Could you check a few things on this drawing? It's one solid part, dimensions in mm from its lowest x, y, z. A direction names the side the tool comes from. Give positions to 0.01 mm unless a question says otherwise; leave off trailing zeros. Loops run counter-clockwise (first coordinate to the right, second up) from the corner with the lowest first, then second, coordinate; pieces in that order, holes last. Notation, with made-up numbers: (76.25, -40) -> (127.25, -40) arc R22 cw to (127.25, -13) -> close; hole circle Ø4 at (28, -11). An arc over 180 degrees is marked (long way). One line per question, with ' | ' between items.
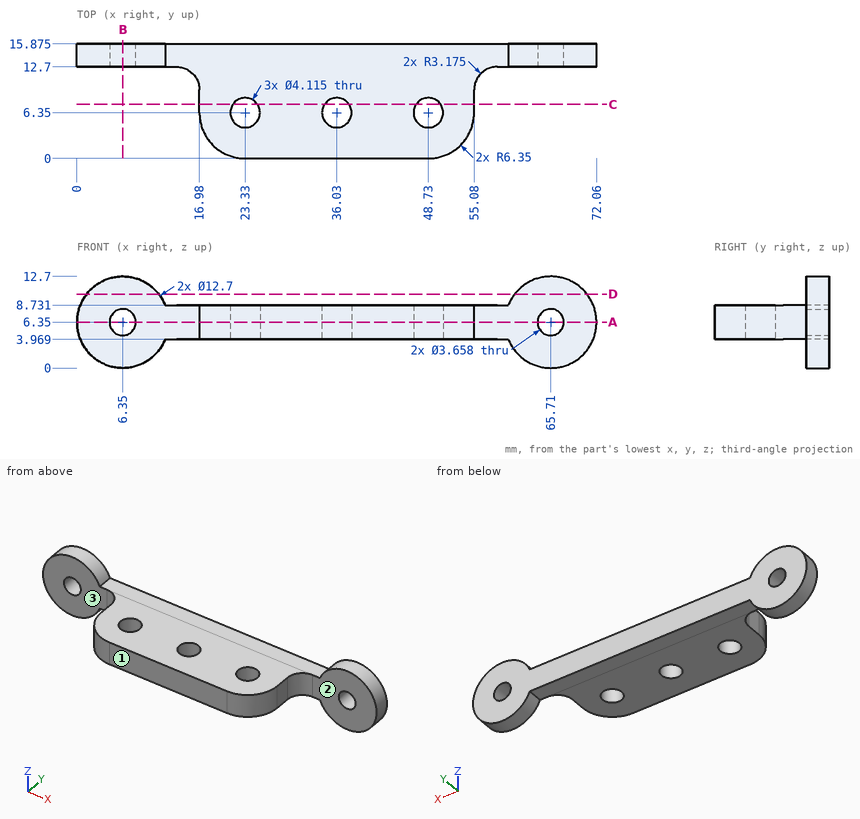
Q1. For pin 1 Ø6 at (x, z) = (61.5, 8) entering from -Y; pin 2 Ø2.5 at (x, y) = (29, 14.5) entering from +Z; pin 3 Ø1.6 at (x, y) = (28, 15) entering from -Z; pin 4 Ø6 at (x, z) = (65.71, 6.35) entering from +Y (3 decimals), each with a flat end and sliding along its axis, tell me the tip position at first contact or that it passes through.
Entries:
pin 1: y = 12.7 | pin 2: z = 8.73 | pin 3: z = 3.97 | pin 4: y = 15.875
Q2. If we section it at B-B (x = 6.35): Write out the boundary of the cut face in (y, z) (1 decimal).
Entries:
outline: (12.7, 0) -> (15.9, 0) -> (15.9, 4.5) -> (12.7, 4.5) -> close; (12.7, 8.2) -> (15.9, 8.2) -> (15.9, 12.7) -> (12.7, 12.7) -> close
Q3. On a 3-axis mill with a long thin cutter (end or side, diameter ignored), from which of +Z, -Z, +X, -X, +Y, -Y can I reach the whole of each face in a straight line? I mean the marked faces 1, 2 and 3. Say none if no direction works.
Entries:
face 1: +Z, -Z, +X, -X, -Y | face 2: +Z, -Z, +X, -Y | face 3: +Z, -Z, -X, -Y
Q4. If we section it at D-D (z = 10.25): Write out the boundary of the cut face in (x, y) (1 decimal).
Entries:
outline: (1.3, 12.7) -> (11.4, 12.7) -> (11.4, 15.9) -> (1.3, 15.9) -> close; (60.7, 12.7) -> (70.7, 12.7) -> (70.7, 15.9) -> (60.7, 15.9) -> close
Q5. If we section it at A-A (z = 6.35): State how many separate pieces and enclosed holes the cut face has.
Entries:
separate pieces: 3 | enclosed holes: 3
Q6. If we section it at C-C (y = 7.5): Write out the boundary of the cut face in (x, z), plus the area to 3 significant figures.
Entries:
outline: (16.98, 3.97) -> (21.62, 3.97) -> (21.62, 8.73) -> (16.98, 8.73) -> close; (25.04, 3.97) -> (34.32, 3.97) -> (34.32, 8.73) -> (25.04, 8.73) -> close; (37.74, 3.97) -> (47.02, 3.97) -> (47.02, 8.73) -> (37.74, 8.73) -> close; (50.44, 3.97) -> (55.08, 3.97) -> (55.08, 8.73) -> (50.44, 8.73) -> close | area: 133 mm²
Q7. If I drill on probe 1 along X at (y, z) = (14, 5) (1 decimal); probe 2 along Y at (x, z) = (65, 10.5) (1 decimal); probe 3 along Z at (x, y) = (32.5, 5.5), over which ranges is the centre line in solid material (lowest first)? Write a range as from..to.
Entries:
probe 1: 0.1..5.1, 7.6..64.5, 66.9..71.9 | probe 2: 12.7..15.9 | probe 3: 3.97..8.73
